Here's how the part is built. I have some questions about the finished solid (model axes, mm). A direction names the side the tool comes from. Give positions to 0.01 mm unless a question says otherwise; leave off trailing zeros. Order: outer loops, then holes, each group sorted by start corner. A loop starts at its lowest first (then second) coordinate and runs counter-clockwise, first axis right, second up. Notation, with made-up numbers: M -30.75,47 L -5.75,47 A14 cw -5.75,53 Z; hole C -26,41 d6. An arc over 180 degrees is marked long. Use one line per item in the form item = value.
from build123d import *

# Parameters (mm, degrees)
CUT_EXTRUDE1_DEPTH = 1.3


with BuildPart() as part:
    # Sketch1 → Revolve1 (revolve)
    with BuildSketch(Plane.XY):
        with BuildLine():
            Line((14.2, 0), (14.2, 1.61))
            Line((14.2, 1.61), (13.81, 2))
            Line((13.81, 2), (2.2, 2))
            Line((2.2, 2), (2.2, 3.8))
            Line((2.2, 3.8), (1.82, 3.8))
            ThreePointArc((1.82, 3.8), (0.762013659, 2.991755338), (0, 1.9))
            Line((0, 1.9), (0, 0))
            Line((0, 0), (14.2, 0))
        make_face()
    revolve(axis=Axis((-2.02471666, 0, 0), (1, 0, 0)))

    # Sketch2 → Cut-Extrude1 (cut)
    with BuildSketch(Plane.ZY):
        Polygon((0.702687556, -1.260969814), (1.44337567, -0.021939633), (0.740688114, 1.239030181), (-0.702687556, 1.260969814), (-1.44337567, 0.021939633), (-0.740688114, -1.239030181), align=None)
    extrude(amount=-CUT_EXTRUDE1_DEPTH, mode=Mode.SUBTRACT)


solid = part.part
Q1. I'm going to push flat-ended pins straight in: pin 1 Ø1.5 at (x, z) = (5.5, 2.5) entering from +Y; pin 2 Ø1 at (x, y) = (7, 2) entering from -Z; pin 3 Ø1.3 at (y, z) = (0, 0.5) entering from -X. Where does each tip first touch, or does it pass through?
Found:
pin_1 = 0.97
pin_2 = -1.32
pin_3 = 1.3
Q2. I want a section at A-A on z = 0. Write out the boundary of the cut face in (x, y), then the cut area to 3 significant figures.
Found:
outline = M 0,-1.9 A4.32 ccw 1.82,-3.8 L 2.2,-3.8 L 2.2,-2 L 13.81,-2 L 14.2,-1.61 L 14.2,1.61 L 13.81,2 L 2.2,2 L 2.2,3.8 L 1.82,3.8 A4.32 ccw 0,1.9 L 0,1.25 L 1.3,1.25 L 1.3,-1.25 L 0,-1.25 Z
area = 58.6 mm²
Q3. On a 3-axis mill with a long thin cutter (end or side, diameter ignored), from which of +Z, -Z, +X, -X, +Y, -Y can I reach the whole of each face in a straight line? I mean faces 4 (the face through (0.64, 0.65, -1.07)), 5 (the face through (14.2, 0, 0)). Say none if no direction works.
Found:
face_4 = -X
face_5 = +Z, -Z, +X, +Y, -Y
Q4. I need wall thicknesses on L1, parallel to Z at x = 4.25, y = 1.25; L2, parallel to Y at x = 10.25, z = -0.5; L3, parallel to X at y = 0, z = 0.75. Which ranges of each line are inside material? Lowest first, please.
Found:
L1 = -1.56 to 1.56
L2 = -1.94 to 1.94
L3 = 1.3 to 14.2
Q5. I want a section at B-B on y = -2.5. Write out the boundary of the cut face in (x, z).
Found:
outline = M 1.82,-2.86 L 2.2,-2.86 L 2.2,2.86 L 1.82,2.86 A3.53 ccw Z
Q6. I want a section at C-C on x = 10.75. Write out the boundary of the cut face in (y, z).
Found:
outline = C 0,0 d4
Q7. Thinking about a two-plate mould opening in Z: for faces 1 (the face through (8, 0, -2)), 2 (the face through (2.2, -2, -2)), 3 (the face through (0.641, 0.6, 1.097)), which applies, +Z half, -Z half, draft (parallel to the pull), parting line (faces both ways), or undercut?
Found:
face_1 = parting line
face_2 = draft
face_3 = undercut
Q8. I want a section at D-D on z = -3. Write out the boundary of the cut face in (x, y).
Found:
outline = M 1.82,-2.33 L 2.2,-2.33 L 2.2,2.33 L 1.82,2.33 A3.12 ccw Z
